```python
from build123d import *

# Parameters (mm, degrees)
CUT_EXTRUDE1_START = -6.35
CUT_EXTRUDE1_DEPTH = 6.35


with BuildPart() as part:
    # Sketch1 → Revolve1 (revolve)
    with BuildSketch(Plane.XY):
        Polygon((0, 0), (0, 15.24), (0, 22.86), (10.16, 22.86), (10.16, 16.51), (12.0396, 16.51), (12.0396, 15.24), (10.0076, 15.24), (10.0076, 0), align=None)
    revolve(axis=Axis((0, 0, 0), (0, 1, 0)))

    # Sketch2 → Cut-Extrude1 (cut)
    with BuildSketch(Plane(origin=(0, 22.86, 0), x_dir=(1, 0, 0), z_dir=(0, 1, 0)).offset(CUT_EXTRUDE1_START)):
        with BuildLine():
            ThreePointArc((5.08, 8.798818102), (0, 10.16), (-5.08, 8.798818102))
            Line((-5.08, 8.798818102), (5.08, 8.798818102))
        make_face()
        with BuildLine():
            Line((-10.16, 0), (-5.08, 8.798818102))
            ThreePointArc((-5.08, 8.798818102), (-8.798818102, 5.08), (-10.16, 0))
        make_face()
        with BuildLine():
            Line((-5.08, -8.798818102), (-10.16, 0))
            ThreePointArc((-10.16, 0), (-8.798818102, -5.08), (-5.08, -8.798818102))
        make_face()
        with BuildLine():
            ThreePointArc((10.16, 0), (8.798818102, 5.08), (5.08, 8.798818102))
            Line((5.08, 8.798818102), (10.16, 0))
        make_face()
        with BuildLine():
            Line((5.08, -8.798818102), (-5.08, -8.798818102))
            ThreePointArc((-5.08, -8.798818102), (0, -10.16), (5.08, -8.798818102))
        make_face()
        with BuildLine():
            ThreePointArc((5.08, -8.798818102), (8.798818102, -5.08), (10.16, 0))
            Line((10.16, 0), (5.08, -8.798818102))
        make_face()
    extrude(amount=CUT_EXTRUDE1_DEPTH, mode=Mode.SUBTRACT)


solid = part.part
```
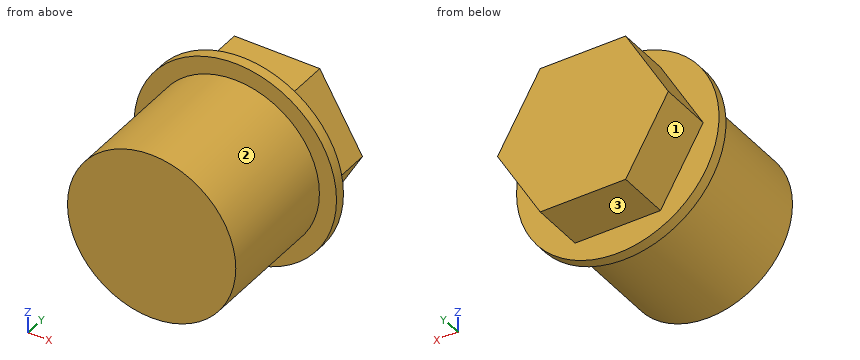
Input: part model. Units: mm. Frame: model coordinates. Face numbers are marked on the shaded views. A direction names the side the tool comes from. Give positions to 0.01 mm unless a question says otherwise; leave off trailing zeros. Order: outer loops, then holes, each group sorted by start corner. A loop starts at its lowest first (then second) coordinate and runs counter-clockwise, first axis right, second up. Notation, with made-up numbers: (88, 6.25) - (139, 6.25) arc R20 cw to (139, 25.25) - close; hole circle Ø1 at (35.25, -19.75). An arc over 180 degrees is marked (long way). Put each result on its own line as item: value.
Item 1: Access query for the marked faces 1, 2 and 3. Directions: +Z, -Z, +X, -X, +Y, -Y. A direction counts if a zero-diameter tool reaches every point of the face in a straight line with its end or side. Return the directions, or none.
Found:
face 1: -Z, -X, +Y
face 2: -Y
face 3: -Z, +X, -X, +Y
Item 2: Section query B-B, the plane y = 17. Return loops of the section in (x, z).
Found:
outline: (-10.16, 0) - (-5.08, -8.8) - (5.08, -8.8) - (10.16, 0) - (5.08, 8.8) - (-5.08, 8.8) - close
Item 3: Section query D-D, the plane y = 11. Return loops of the section in (x, z), then the cut area to 3 significant figures.
Found:
outline: circle Ø20.02 at (0, 0)
area: 315 mm^2
Item 4: Contact query for flat-ended pins moving along their axis: pin 1 (8 mm diameter, centred on x = 9, z = -8, fed in from +Y); pin 2 (5 mm diameter, centred on x = 0.5, y = 19.5, fed in from -Z); pin 3 (4 mm diameter, centred on y = 8.5, z = 7, fed in from -X); pin 4 (2 mm diameter, centred on x = 5, y = 15.5, fed in from +Z). Output: stop coordinate, or through.
Found:
pin 1: stops at y = 22.86
pin 2: stops at z = -8.8
pin 3: stops at x = -8.67
pin 4: stops at z = 11.36
Item 5: Section query C-C, the plane z = 2.5. Return loops of the section in (x, y).
Found:
outline: (-11.78, 15.24) - (-9.69, 15.24) - (-9.69, 0) - (9.69, 0) - (9.69, 15.24) - (11.78, 15.24) - (11.78, 16.51) - (8.72, 16.51) - (8.72, 22.86) - (-8.72, 22.86) - (-8.72, 16.51) - (-11.78, 16.51) - close
Item 6: Section query A-A, the plane x = 0. Return loops of the section in (y, z).
Found:
outline: (0, -10.01) - (15.24, -10.01) - (15.24, -12.04) - (16.51, -12.04) - (16.51, -8.8) - (22.86, -8.8) - (22.86, 8.8) - (16.51, 8.8) - (16.51, 12.04) - (15.24, 12.04) - (15.24, 10.01) - (0, 10.01) - close
Item 7: Ray query, L1, parallel to Z at x = -0.25, y = 6; L2, parallel to Y at x = -9, z = -3; L3, parallel to Z at x = -1.5, y = 20.25. Return the intervals inside material, ascending. Write a range as from..to.
Found:
L1: z = -10..10
L2: y = 0..16.51
L3: z = -8.8..8.8
